Source: CAD feature listing. Evaluate the final solid. Frame: model axes, mm. A direction names the side the tool comes from. Coordinates: 2 decimals unless noted, no trailing zeros. Write each loop counter-clockwise with the first axis right and the second up, starting at its lowest first coordinate (ties: lowest second). Pieces come first, ordered by that corner, then holes. Notation, with made-up numbers: (-40, 77.5) -> (6, 77.5) arc R14 ccw to (6, 102.5) -> close; hole circle Ø5 at (34, 72). An arc over 180 degrees is marked (long way). One line per item, written item: value. Start each with the question number.
1. Line query: line 1 (X direction, y = 0.7, z = 16.5); line 2 (Y direction, x = 39, z = -14); line 3 (Y direction, x = -24.5, z = 5). Output: solid intervals per line, ascending.
2. Section query B-B, the plane x = -8.5. Output: boundary loops of the cut face in (y, z), and give its area (3 significant figures).
3. Section query C-C, the plane z = -10. Output: boundary loops of the cut face in (x, y).
4. Section query A-A, the plane x = -48.5. Output: boundary loops of the cut face in (y, z).
5. Mould query, pull axis Z, two halves, no side actions, for faces 1 (the flat face through (39.6, 5, -16.4)), 2 (the flat face through (44, 3, 13)), 3 (the flat face through (8, 3, -18)). Classes: released by +Z, released by -Z, zero draft, split by the parting line, or undercut.
6. Section query D-D, the plane y = 12.5. Output: boundary loops of the cut face in (x, z), and give its area (3 significant figures).
7. Access query for faces 4 (the flat face through (-44, 11.5, 8)), 5 (the flat face through (-42, 4, 12.5)), 6 (the flat face through (41, 3, -18)), 7 (the flat face through (8, 3, 16)), 8 (the flat face through (5, 3, 13)). Directions: +Z, -Z, +X, -X, +Y, -Y. A direction counts if a zero-diameter tool reaches every point of the face in a straight line with its end or side. Return the directions, or none.
8. First-contact query: P1, Ø1.8, axis at x = 7.5, y = 3, coming from the +Z side; P2, Ø1, axis at y = 2.5, z = 14, coming from the +X side; P3, Ø1.8, axis at x = 7, z = -1, coming from the +Y side. Flat tips, straight axial feed; report the tip coordinate or a pass-through.
from build123d import *
from build123d.topology import SkipClean

# Parameters (mm, degrees)
SKETCH1_W           = 103
SKETCH1_H           = 38
BOSS_EXTRUDE1_DEPTH = 1.5
SKETCH2_R           = 1.5
CUT_EXTRUDE1_DEPTH  = 55.913568451
SKETCH3_R           = 1.5
BOSS_EXTRUDE2_DEPTH = 9.5
SKETCH5_W           = 6
SKETCH5_H           = 6
BOSS_EXTRUDE3_DEPTH = 3.5
BOSS_EXTRUDE4_DEPTH = 20
SKETCH7_R           = 3
BOSS_EXTRUDE5_DEPTH = 13
SKETCH8_R           = 3.5
BOSS_EXTRUDE6_DEPTH = 10
SKETCH9_W           = 12
SKETCH9_H           = 13
BOSS_EXTRUDE7_DEPTH = 5


with BuildPart() as part:
    # Sketch1 → Boss-Extrude1 (new body)
    with BuildSketch(Plane(origin=(0, 0, 0), x_dir=(1, 0, 0), z_dir=(0, 1, 0))):
        Rectangle(SKETCH1_W, SKETCH1_H)
    extrude(amount=BOSS_EXTRUDE1_DEPTH)

    # Sketch2 → Cut-Extrude1 (cut, through all)
    with BuildSketch(Plane(origin=(0, 1.5, 0), x_dir=(1, 0, 0), z_dir=(0, 1, 0))):
        with Locations(Location((-48.5, 16.5, 0), (0, 0, 270))):
            Circle(SKETCH2_R)
        with Locations(Location((-48.5, -16.5, 0), (0, 0, 270))):
            Circle(SKETCH2_R)
        with Locations(Location((48.5, -16.5, 0), (0, 0, 270))):
            Circle(SKETCH2_R)
        with Locations(Location((48.5, 16.5, 0), (0, 0, 270))):
            Circle(SKETCH2_R)
    extrude(amount=-CUT_EXTRUDE1_DEPTH, mode=Mode.SUBTRACT)

    # Sketch3 → Boss-Extrude2 (add)
    with BuildSketch(Plane(origin=(0, 1.5, 0), x_dir=(1, 0, 0), z_dir=(0, 1, 0))):
        with Locations(Location((41, 15, 0), (0, 0, 270))):
            Circle(SKETCH3_R)
        with Locations(Location((41, 1, 0), (0, 0, 270))):
            Circle(SKETCH3_R)
        with Locations(Location((41, -13, 0), (0, 0, 270))):
            Circle(SKETCH3_R)
        with Locations(Location((24.5, 1, 0), (0, 0, 270))):
            Circle(SKETCH3_R)
        with Locations(Location((8, 1, 0), (0, 0, 270))):
            Circle(SKETCH3_R)
        with Locations(Location((8, 15, 0), (0, 0, 270))):
            Circle(SKETCH3_R)
        with Locations(Location((8, -13, 0), (0, 0, 270))):
            Circle(SKETCH3_R)
        with Locations(Location((-8.5, 1, 0), (0, 0, 270))):
            Circle(SKETCH3_R)
        with Locations(Location((-41.5, 10, 0), (0, 0, 270))):
            Circle(SKETCH3_R)
    extrude(amount=BOSS_EXTRUDE2_DEPTH)

    # Sketch5 → Boss-Extrude3 (add)
    with BuildSketch(Plane(origin=(0, 1.5, 0), x_dir=(1, 0, 0), z_dir=(0, 1, 0))):
        with Locations((8, 15)):
            Rectangle(SKETCH5_W, SKETCH5_H)
        with Locations((24.5, 1)):
            Rectangle(SKETCH5_W, SKETCH5_H)
        with Locations((8, 1)):
            Rectangle(SKETCH5_W, SKETCH5_H)
        with Locations((-8.5, 1)):
            Rectangle(SKETCH5_W, SKETCH5_H)
        with Locations((8, -13)):
            Rectangle(SKETCH5_W, SKETCH5_H)
        with Locations((41, -13)):
            Rectangle(SKETCH5_W, SKETCH5_H)
        with Locations((41, 1)):
            Rectangle(SKETCH5_W, SKETCH5_H)
        with Locations((41, 15)):
            Rectangle(SKETCH5_W, SKETCH5_H)
        with Locations((-41.5, 10)):
            Rectangle(SKETCH5_W, SKETCH5_H)
    extrude(amount=BOSS_EXTRUDE3_DEPTH)

    # Sketch6 → Boss-Extrude4 (add)
    with BuildSketch(Plane(origin=(0, 1.5, 0), x_dir=(1, 0, 0), z_dir=(0, 1, 0))):
        with BuildLine():
            Line((-38.671572875, -7), (-44.328427125, -7))
            ThreePointArc((-44.328427125, -7), (-41.5, -3), (-38.671572875, -7))
        make_face()
    extrude(amount=BOSS_EXTRUDE4_DEPTH)

    # Sketch7 → Boss-Extrude5 (add)
    with SkipClean():  # the faces are left unmerged after this step: merging them gives an invalid solid
        with BuildSketch(Plane(origin=(0, 1.5, 0), x_dir=(1, 0, 0), z_dir=(0, 1, 0))):
            with Locations(Location((-41.5, -6, 0), (0, 0, 340.528779366))):
                Circle(SKETCH7_R)
        extrude(amount=BOSS_EXTRUDE5_DEPTH)

    # Sketch8 → Boss-Extrude6 (add)
    with SkipClean():  # the faces are left unmerged after this step: merging them gives an invalid solid
        with BuildSketch(Plane(origin=(0, 1.5, 0), x_dir=(1, 0, 0), z_dir=(0, 1, 0))):
            with Locations(Location((-41.5, -6, 0), (0, 0, 270))):
                Circle(SKETCH8_R)
        extrude(amount=BOSS_EXTRUDE6_DEPTH)

    # Sketch9 → Boss-Extrude7 (add)
    with SkipClean():  # the faces are left unmerged after this step: merging them gives an invalid solid
        with BuildSketch(Plane(origin=(0, 1.5, 0), x_dir=(1, 0, 0), z_dir=(0, 1, 0))):
            with Locations((-41.5, -6)):
                Rectangle(SKETCH9_W, SKETCH9_H)
        extrude(amount=BOSS_EXTRUDE7_DEPTH)


solid = part.part
Computed values:
1. line 1: x = -51.5 to -50, -47 to 47, 50 to 51.5
1. line 2: y = 0 to 5
1. line 3: y = 0 to 1.5
2. outline: (0, -19) -> (1.5, -19) -> (1.5, -4) -> (5, -4) -> (5, -2.5) -> (11, -2.5) -> (11, 0.5) -> (5, 0.5) -> (5, 2) -> (1.5, 2) -> (1.5, 19) -> (0, 19) -> close
2. area: 96.0 mm²
3. outline: (-51.5, 0) -> (51.5, 0) -> (51.5, 1.5) -> (-38.5, 1.5) -> (-38.5, 5) -> (-40, 5) -> (-40, 11) -> (-43, 11) -> (-43, 5) -> (-44.5, 5) -> (-44.5, 1.5) -> (-51.5, 1.5) -> close
4. outline: (0, -19) -> (1.5, -19) -> (1.5, -18) -> (0, -18) -> close; (0, -15) -> (1.5, -15) -> (1.5, 15) -> (0, 15) -> close; (0, 18) -> (1.5, 18) -> (1.5, 19) -> (0, 19) -> close
5. face 1: undercut
5. face 2: zero draft
5. face 3: released by -Z
6. outline: circle Ø6 at (-41.5, 6)
6. area: 28.3 mm²
7. face 4: +Y
7. face 5: +Z, -X, +Y
7. face 6: -Z, +X, -X, +Y
7. face 7: +Z, +X, -X, +Y
7. face 8: +Z, -Z, +Y
8. P1: stops at z = 16
8. P2: stops at x = 44
8. P3: stops at y = 11
